Source: three-view drawing plus pictorial views. Frame: mm from the lowest corner of the part. A direction names the side the tool comes from. Coordinates: 2 decimals unless noted, no trailing zeros. Order: outer loops, then holes, each group sorted by start corner. A loop starts at its lowest first (then second) coordinate and runs counter-clockwise, first axis right, second up. Notation, with made-up numbers: (85, 89.25) -> (143, 89.25) arc R16 ccw to (143, 101.25) -> close; hole circle Ø1 at (-37, 7.25). An arc over 180 degrees is marked (long way). One line per question, with ' | ' between items.
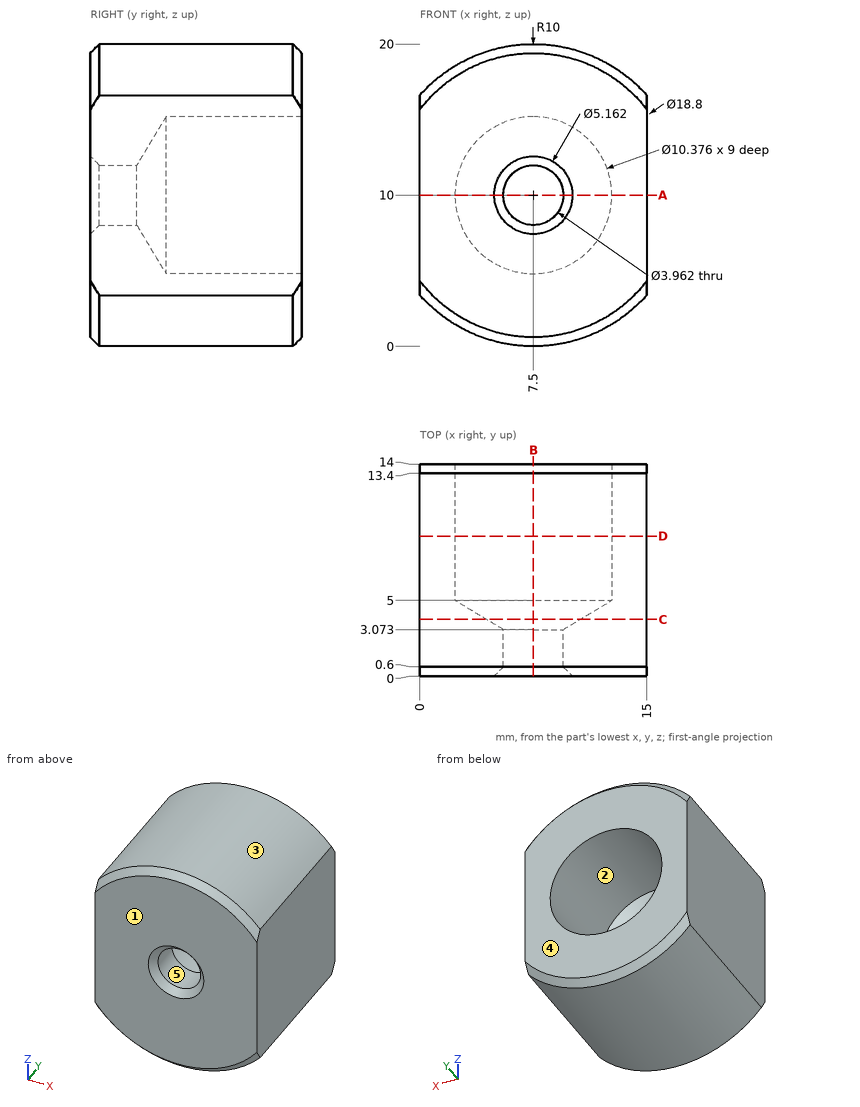
1. Cut plane B-B, the plane x = 7.5. Return loops of the section in (y, z).
Recorded:
outline: (0, 0.6) -> (0.6, 0) -> (13.4, 0) -> (14, 0.6) -> (14, 4.81) -> (5, 4.81) -> (3.07, 8.02) -> (0.6, 8.02) -> (0, 7.42) -> close; (0, 12.58) -> (0.6, 11.98) -> (3.07, 11.98) -> (5, 15.19) -> (14, 15.19) -> (14, 19.4) -> (13.4, 20) -> (0.6, 20) -> (0, 19.4) -> close
2. Cut plane A-A, the plane z = 10. Return loops of the section in (x, y).
Recorded:
outline: (0, 0) -> (4.92, 0) -> (5.52, 0.6) -> (5.52, 3.07) -> (2.31, 5) -> (2.31, 14) -> (0, 14) -> close; (9.48, 0.6) -> (10.08, 0) -> (15, 0) -> (15, 14) -> (12.69, 14) -> (12.69, 5) -> (9.48, 3.07) -> close
3. Pin query (flat end, axial travel): pin 1 Ø5 at (x, y) = (6, 9.5) entering from +Z; pin 2 Ø1 at (x, z) = (5, 11.5) entering from +Y (1 decimal); pin 3 Ø8.5 at (x, z) = (7.5, 10) entering from +Y; pin 4 Ø1.5 at (x, z) = (5, 13) entering from +Y. Return the tip coordinate at first contact, or that it passes through.
Recorded:
pin 1: stops at z = 20 | pin 2: stops at y = 3.9 | pin 3: stops at y = 4.44 | pin 4: stops at y = 4.68
4. Access query for the marked faces 1 and 2. Directions: +Z, -Z, +X, -X, +Y, -Y. A direction counts if a zero-diameter tool reaches every point of the face in a straight line with its end or side. Return the directions, or none.
Recorded:
face 1: +Z, -Z, +X, -X, -Y | face 2: +Y
5. Mould query, pull axis Z, two halves, no side actions, for the marked faces 3, 4 and 5. Classes: released by +Z, released by -Z, zero draft, split by the parting line, or undercut.
Recorded:
face 3: released by +Z | face 4: zero draft | face 5: undercut
6. Cut plane C-C, the plane y = 3.75. Return loops of the section in (x, z) (1 decimal).
Recorded:
outline: (0, 3.4) arc R10 ccw to (15, 3.4) -> (15, 16.6) arc R10 ccw to (0, 16.6) -> close; hole circle Ø6.2 at (7.5, 10)
7. Ray query, line 1 (Z direction, x = 7.5, y = 11.75); line 2 (X direction, y = 9, z = 10.25); line 3 (X direction, y = 1.4, z = 10). Return the intervals inside material, ascending. Write a range as [from, to].
Recorded:
line 1: z = [0, 4.81], [15.19, 20] | line 2: x = [0, 2.32], [12.68, 15] | line 3: x = [0, 5.52], [9.48, 15]
8. Cut plane D-D, the plane y = 9.25. Return loops of the section in (x, z) (1 decimal).
Recorded:
outline: (0, 3.4) arc R10 ccw to (15, 3.4) -> (15, 16.6) arc R10 ccw to (0, 16.6) -> close; hole circle Ø10.4 at (7.5, 10)
